CAD build for the part. Positions are in the model's coordinates, mm. A direction names the side the tool comes from. Give positions to 0.01 mm unless a question says otherwise; leave off trailing zeros. Order: outer loops, then holes, each group sorted by start corner. A loop starts at its lowest first (then second) coordinate and runs counter-clockwise, first axis right, second up. Notation, with made-up numbers: (54.25, 13.25) -> (105.25, 13.25) arc R12 ccw to (105.25, 31.25) -> close; hole circle Ø2 at (-7.5, 86.25). An arc over 180 degrees is marked (long way). Use one line per item in the form item = value. Start each with the question number.
1) Mould opens along X. For faces 3 (the face through (7, -1.8, 3)), 4 (the face through (7.24, 38.783, 1.734)), 5 (the face through (7, -1, 2.595)), 6 (the face through (11.5, 35, 2)) say: pulls with the +X half, pulls with the -X half, needs draft (parallel to the pull), parting line crosses it, or undercut.
2) Cut at C-C, the plane z = 0.7. Give the cut face in (x, y) (3 decimals), and give its area (3 significant figures).
3) Tool access for faces 1 (the face through (7.4, -0.2, 2.8)), 2 (the face through (7, 15, 4.6)): list every direction of +Z, -Z, +X, -X, +Y, -Y with a clear straight run to the whole face (end or side of a thin tool).
4) Cut at B-B, the plane x = 7.5. Give the cut face in (y, z) (3 decimals).
5) Cut at D-D, the plane y = 24.5. Give the cut face in (x, z).
6) Drop flat-ended pins along their axis: P1, Ø2, axis at x = 4, y = 6.5, coming from the -Z side; P2, Ø8.5, axis at x = 8, y = 19, coming from the -Z side; P3, Ø1, axis at x = 2, y = 7, coming from the -Z side; P4, Ø2.5, axis at x = 7.5, y = 36.8, coming from the +Z side. Give the stop position or say it passes through.
7) Probe line 1 (Y direction, x = 2, z = 2.6); line 2 (X direction, y = 29, z = 2.6); line 3 (X direction, y = 29, z = 3.05). List the from-to ranges inside material, lowest first.
8) Cut at A-A, the plane y = 36.8. Give the cut face in (x, z), and give its area (4 significant figures).
from build123d import *

# Parameters (mm, degrees)
SKETCH_W           = 15.4
SKETCH_H           = 31.4
PAD_DEPTH          = 3
THICKNESS_T        = 1.6
SKETCH001_W        = 18.6
SKETCH001_H        = 34.6
SKETCH001_W_2      = 17
SKETCH001_H_2      = 33
PAD001_DEPTH       = 0.7
SKETCH002_W        = 8.45
SKETCH002_H        = 3.295
POCKET_DEPTH       = 5
SKETCH003_R        = 2
PAD002_DEPTH       = 1.49
SKETCH004_R        = 1
POCKET001_DEPTH    = 2.1
SKETCH009_W        = 8
SKETCH009_H        = 5.3
PAD006_DEPTH       = 8
SKETCH010_R        = 2
POCKET002_DEPTH    = 5.301
FILLET_R           = 3
CHAMFER_SIZE       = 0.5
CHAMFER001_SIZE    = 0.5
CHAMFER005_1_SIZE2 = 0.4
CHAMFER005_1_SIZE  = 0.2
CHAMFER005_2_SIZE2 = 0.4
CHAMFER005_2_SIZE  = 0.2
CHAMFER005_3_SIZE2 = 0.4
CHAMFER005_3_SIZE  = 0.2
CHAMFER005_4_SIZE2 = 0.4
CHAMFER005_4_SIZE  = 0.2


with BuildPart() as part:
    # Sketch (on Face2746 of Binder) → Pad (new body)
    with BuildSketch(Plane(origin=(0, 0, 0), x_dir=(1, 0, 0), z_dir=(0, 0, -1))):
        with Locations((7.5, -15.5)):
            Rectangle(SKETCH_W, SKETCH_H)
    extrude(amount=-PAD_DEPTH)

    # Thickness
    thickness_openings = [part.faces().sort_by_distance(p)[0] for p in [
        (7.5, 15.5, 0),
    ]]
    offset(amount=THICKNESS_T, openings=thickness_openings, kind=Kind.INTERSECTION)

    # Sketch001 (on Face6 of Thickness) → Pad001 (join)
    with BuildSketch(Plane(origin=(0, 0, 0), x_dir=(1, 0, 0), z_dir=(0, 0, -1))):
        with Locations((7.5, -15.5)):
            Rectangle(SKETCH001_W, SKETCH001_H)
        with Locations((7.5, -15.5)):
            Rectangle(SKETCH001_W_2, SKETCH001_H_2, mode=Mode.SUBTRACT)
    extrude(amount=PAD001_DEPTH)

    # Sketch002 (on Face16 of Pad001) → Pocket (cut)
    with BuildSketch(Plane.XZ.offset(1.8)):
        with Locations((7.5, 0.9475)):
            Rectangle(SKETCH002_W, SKETCH002_H)
    extrude(amount=-POCKET_DEPTH, mode=Mode.SUBTRACT)

    # Sketch003 (on Face18 of Pocket) → Pad002 (join)
    with BuildSketch(Plane(origin=(0, 0, 3), x_dir=(1, 0, 0), z_dir=(0, 0, -1))):
        with Locations((2, -7)):
            Circle(SKETCH003_R)
        with Locations((13, -7)):
            Circle(SKETCH003_R)
        with Locations((2, -29)):
            Circle(SKETCH003_R)
        with Locations((13, -29)):
            Circle(SKETCH003_R)
    extrude(amount=PAD002_DEPTH)

    # Sketch004 (on Face25 of Pad002) → Pocket001 (cut)
    with BuildSketch(Plane(origin=(0, 0, 1.51), x_dir=(1, 0, 0), z_dir=(0, 0, -1))):
        with Locations((2, -7)):
            Circle(SKETCH004_R)
        with Locations((13, -7)):
            Circle(SKETCH004_R)
        with Locations((2, -29)):
            Circle(SKETCH004_R)
        with Locations((13, -29)):
            Circle(SKETCH004_R)
    extrude(amount=-POCKET001_DEPTH, mode=Mode.SUBTRACT)

    # Sketch009 (on Face3 of Pocket001) → Pad006 (join)
    with BuildSketch(Plane(origin=(0, 32.8, 0), x_dir=(-1, 0, 0), z_dir=(0, 1, 0))):
        with Locations((-7.5, 1.95)):
            Rectangle(SKETCH009_W, SKETCH009_H)
    extrude(amount=PAD006_DEPTH)

    # Sketch010 (on Face39 of Pad006) → Pocket002 (cut, through all)
    with BuildSketch(Plane.XY.offset(4.6)):
        with Locations((7.5, 36.8)):
            Circle(SKETCH010_R)
    extrude(amount=-POCKET002_DEPTH, mode=Mode.SUBTRACT)

    # Fillet
    fillet_edges = [part.edges().sort_by_distance(p)[0] for p in [
        (3.5, 40.8, 1.95),
        (11.5, 40.8, 1.95),
    ]]
    fillet(fillet_edges, radius=FILLET_R)

    # Chamfer
    chamfer_edges = [part.edges().sort_by_distance(p)[0] for p in [
        (-1.8, 32.8, 1.95),
        (16.8, 32.8, 1.95),
        (16.8, -1.8, 1.95),
        (-1.8, -1.8, 1.95),
        (16, -1, -0.35),
        (16, 32, -0.35),
        (-1, 32, -0.35),
        (-1, -1, -0.35),
    ]]
    chamfer(chamfer_edges, length=CHAMFER_SIZE)

    # Chamfer001
    chamfer001_edges = [part.edges().sort_by_distance(p)[0] for p in [
        (13.9, 32.8, 4.6),
        (16.55, 32.55, 4.6),
        (11.5, 35.3, 4.6),
        (16.8, 15.5, 4.6),
        (10.62132, 39.92132, 4.6),
        (16.55, -1.55, 4.6),
        (7.5, 40.8, 4.6),
        (7.5, -1.8, 4.6),
        (4.37868, 39.92132, 4.6),
        (-1.55, -1.55, 4.6),
        (3.5, 35.3, 4.6),
        (-1.8, 15.5, 4.6),
        (1.1, 32.8, 4.6),
        (-1.55, 32.55, 4.6),
        (5.5, 36.8, 4.6),
        (11.5, 35.3, -0.7),
        (10.62132, 39.92132, -0.7),
        (7.5, 40.8, -0.7),
        (4.37868, 39.92132, -0.7),
        (3.5, 35.3, -0.7),
    ]]
    chamfer(chamfer001_edges, length=CHAMFER001_SIZE)

    # Chamfer005 1
    chamfer005_1_edges = [part.edges().sort_by_distance(p)[0] for p in [
        (1, 7, 1.51),
    ]]
    chamfer005_1_side = part.faces().sort_by_distance((0.056569, 7, 1.51))[0]
    chamfer(chamfer005_1_edges, length=CHAMFER005_1_SIZE, length2=CHAMFER005_1_SIZE2, reference=chamfer005_1_side)

    # Chamfer005 2
    chamfer005_2_edges = [part.edges().sort_by_distance(p)[0] for p in [
        (12, 7, 1.51),
    ]]
    chamfer005_2_side = part.faces().sort_by_distance((11.056569, 7, 1.51))[0]
    chamfer(chamfer005_2_edges, length=CHAMFER005_2_SIZE, length2=CHAMFER005_2_SIZE2, reference=chamfer005_2_side)

    # Chamfer005 3
    chamfer005_3_edges = [part.edges().sort_by_distance(p)[0] for p in [
        (1, 29, 1.51),
    ]]
    chamfer005_3_side = part.faces().sort_by_distance((0.056569, 29, 1.51))[0]
    chamfer(chamfer005_3_edges, length=CHAMFER005_3_SIZE, length2=CHAMFER005_3_SIZE2, reference=chamfer005_3_side)

    # Chamfer005 4
    chamfer005_4_edges = [part.edges().sort_by_distance(p)[0] for p in [
        (12, 29, 1.51),
    ]]
    chamfer005_4_side = part.faces().sort_by_distance((11.056569, 29, 1.51))[0]
    chamfer(chamfer005_4_edges, length=CHAMFER005_4_SIZE, length2=CHAMFER005_4_SIZE2, reference=chamfer005_4_side)


solid = part.part
Result:
q1.face_3 = needs draft
q1.face_4 = undercut
q1.face_5 = undercut
q1.face_6 = pulls with the +X half
q2.outline = (-1.8, -1.3) -> (-1.3, -1.8) -> (3.275, -1.8) -> (3.275, -0.2) -> (-0.2, -0.2) -> (-0.2, 31.2) -> (15.2, 31.2) -> (15.2, -0.2) -> (11.725, -0.2) -> (11.725, -1.8) -> (16.3, -1.8) -> (16.8, -1.3) -> (16.8, 32.3) -> (16.3, 32.8) -> (11.5, 32.8) -> (11.5, 37.8) arc R3 ccw to (8.5, 40.8) -> (6.5, 40.8) arc R3 ccw to (3.5, 37.8) -> (3.5, 32.8) -> (-1.3, 32.8) -> (-1.8, 32.3) -> close; hole circle Ø4 at (7.5, 36.8)
q2.area = 194 mm²
q3.face_1 = -Z
q3.face_2 = +Z, +X, -X, +Y, -Y
q4.outline = (-1.8, 2.595) -> (-0.2, 2.595) -> (-0.2, 3) -> (31.2, 3) -> (31.2, 0) -> (32, 0) -> (32, -0.7) -> (34.8, -0.7) -> (34.8, 4.1) -> (34.3, 4.6) -> (-1.3, 4.6) -> (-1.8, 4.1) -> close; (38.8, -0.7) -> (40.3, -0.7) -> (40.8, -0.2) -> (40.8, 4.1) -> (40.3, 4.6) -> (39.3, 4.6) -> (38.8, 4.1) -> close
q5.outline = (-1.8, -0.7) -> (-1, -0.7) -> (-1, 0) -> (-0.2, 0) -> (-0.2, 3) -> (15.2, 3) -> (15.2, 0) -> (16, 0) -> (16, -0.7) -> (16.8, -0.7) -> (16.8, 4.1) -> (16.3, 4.6) -> (-1.3, 4.6) -> (-1.8, 4.1) -> close
q6.P1 = 1.51
q6.P2 = 3
q6.P3 = 3.61
q6.P4 = through
q7.line_1 = -1.8 to -0.2, 5 to 6, 8 to 9, 27 to 28, 30 to 31, 31.2 to 32.8
q7.line_2 = -1.8 to -0.2, 0 to 1, 3 to 4, 11 to 12, 14 to 15, 15.2 to 16.8
q7.line_3 = -1.8 to 1, 3 to 12, 14 to 16.8
q8.outline = (3.5, -0.2) -> (4, -0.7) -> (5.5, -0.7) -> (5.5, 4.1) -> (5, 4.6) -> (4, 4.6) -> (3.5, 4.1) -> close; (9.5, -0.7) -> (11, -0.7) -> (11.5, -0.2) -> (11.5, 4.1) -> (11, 4.6) -> (10, 4.6) -> (9.5, 4.1) -> close
q8.area = 20.45 mm²
